Here's how the part is built. I have some questions about the finished solid (model axes, mm). A direction names the side the tool comes from. Round coordinates to 2 decimals unless told otherwise and drop trailing zeros. Loops run counter-clockwise (first coordinate to the right, second up) from the corner with the lowest first, then second, coordinate; pieces in that order, holes last. Notation, with made-up numbers: (26, 21.5) -> (47, 21.5) arc R16 ccw to (47, 28.5) -> close; hole circle Ø3 at (-11, 49.5). An arc over 180 degrees is marked (long way). Use one line per item in the form item = value. Start each with the question number.
Item 1: If we section it at D-D (y = 17.5): Write out the boundary of the cut face in (x, z), then the cut area to 3 significant figures.
Item 2: If we section it at A-A (x = 5.5): Write out the boundary of the cut face in (y, z), then the cut area to 3 significant figures.
Item 3: If we section it at B-B (y = 3): Write out the boundary of the cut face in (x, z), then the cut area to 3 significant figures.
Item 4: Thinking about a two-plate mould opening in Z: for faces 4 (the face through (5, 28, -10.5)), 5 (the face through (0, 13, 0)), 6 (the face through (7, 20, 16.5)), which applies, released by +Z, released by -Z, zero draft, split by the parting line, or undercut?
Item 5: If I drill on L1, parallel to Y at x = 7, z = -12.7; L2, parallel to Z at x = 6.5, y = 21.5; L3, parallel to Y at x = 7, z = 16, over which ranges is the centre line in solid material (lowest first)? Write a range as [from, to].
Item 6: I'm going to push flat-ended pins straight in: pin 1 Ø4 at (x, z) = (12.5, 12.5) entering from +Y; pin 2 Ø8 at (y, z) = (6, -8.5) entering from -X; pin 3 Ø5 at (x, y) = (7, 33) entering from -Z; pin 4 Ø3.5 at (x, z) = (11, 0) entering from +Y. Where does each tip first touch, or does it pass through?
Item 7: For faces 1 (the face through (7, 0, 0)), 2 (the face through (6.9, 29.7, 15.5)), 3 (the face through (7, 15, 0)), which set-ups out of +Z, -Z, +X, -X, +Y, -Y let a thin tool reach every point of the face, with its end or its side?
Item 8: If we section it at C-C (x = 3): Write out the boundary of the cut face in (y, z), then the cut area to 3 significant figures.
```python
from build123d import *

# Parameters (mm, degrees)
EXTRUDE_1_DEPTH     = 14
FILLET_1_R          = 7
CUT_EXTRUDE_START   = -1
SKETCH_7_R          = 5
CUT_EXTRUDE_1_DEPTH = 31
SKETCH_8_R          = 3.1
CUT_EXTRUDE_2_DEPTH = 35
CUT_EXTRUDE_START_2 = 2
SKETCH_10_R         = 1.5
CUT_EXTRUDE_3_DEPTH = 20


with BuildPart() as part:
    # 草图4 → 凸台-拉伸1 (new body)
    with BuildSketch(Plane(origin=(0, 0, 0), x_dir=(0, 0, -1), z_dir=(1, 0, 0))):
        with BuildLine():
            Line((0, 0), (16.5, 0))
            Line((16.5, 0), (16.5, 40))
            Line((16.5, 40), (10.5, 40))
            Line((10.5, 40), (10.5, 20))
            ThreePointArc((10.5, 20), (9.035533906, 16.464466094), (5.5, 15))
            Line((5.5, 15), (-5.5, 15))
            ThreePointArc((-5.5, 15), (-9.035533906, 16.464466094), (-10.5, 20))
            Line((-10.5, 20), (-10.5, 40))
            Line((-10.5, 40), (-16.5, 40))
            Line((-16.5, 40), (-16.5, 0))
            Line((-16.5, 0), (0, 0))
        make_face()
    extrude(amount=EXTRUDE_1_DEPTH)

    # 圆角1
    fillet_1_edges = [part.edges().sort_by_distance(p)[0] for p in [
        (0, 40, 13.5),
        (0, 40, -13.5),
        (14, 40, -13.5),
        (14, 40, 13.5),
    ]]
    fillet(fillet_1_edges, radius=FILLET_1_R - 0.0001)  # a hair under: the kernel refuses the full size

    # 草图7 → 切除-拉伸1 (cut)
    with BuildSketch(Plane.XY.offset(16.5).offset(CUT_EXTRUDE_START)):
        with Locations((7, 33)):
            Circle(SKETCH_7_R)
    extrude(amount=-CUT_EXTRUDE_1_DEPTH, mode=Mode.SUBTRACT)

    # 草图8 → 切除-拉伸2 (cut)
    with BuildSketch(Plane.XY.offset(16.5)):
        with Locations((7, 33)):
            Circle(SKETCH_8_R)
    extrude(amount=-CUT_EXTRUDE_2_DEPTH, mode=Mode.SUBTRACT)

    # 草图10 → 切除-拉伸3 (cut)
    with BuildSketch(Plane(origin=(0, 15, 0), x_dir=(1, 0, 0), z_dir=(0, 1, 0)).offset(CUT_EXTRUDE_START_2)):
        with Locations(Location((3, 0, 0), (0, 0, 270))):
            Circle(SKETCH_10_R)
        with Locations(Location((11, 0, 0), (0, 0, 270))):
            Circle(SKETCH_10_R)
    extrude(amount=-CUT_EXTRUDE_3_DEPTH, mode=Mode.SUBTRACT)


solid = part.part
```
Values found:
q1.outline = (0, -16.5) -> (14, -16.5) -> (14, -9.83) -> (0, -9.83) -> close; (0, 9.83) -> (14, 9.83) -> (14, 16.5) -> (0, 16.5) -> close
q1.area = 187 mm2
q2.outline = (0, -16.5) -> (30.29, -16.5) -> (30.29, -15.5) -> (28.23, -15.5) -> (28.23, -10.5) -> (20, -10.5) arc R5 cw to (15, -5.5) -> (15, 5.5) arc R5 cw to (20, 10.5) -> (28.23, 10.5) -> (28.23, 15.5) -> (30.29, 15.5) -> (30.29, 16.5) -> (0, 16.5) -> close; (35.71, -16.5) -> (39.84, -16.5) -> (39.84, -10.5) -> (37.77, -10.5) -> (37.77, -15.5) -> (35.71, -15.5) -> close; (35.71, 15.5) -> (37.77, 15.5) -> (37.77, 10.5) -> (39.84, 10.5) -> (39.84, 16.5) -> (35.71, 16.5) -> close
q2.area = 698 mm2
q3.outline = (0, -16.5) -> (14, -16.5) -> (14, 16.5) -> (0, 16.5) -> close; hole circle Ø3 at (3, 0); hole circle Ø3 at (11, 0)
q3.area = 448 mm2
q4.face_4 = undercut
q4.face_5 = zero draft
q4.face_6 = released by +Z
q5.L1 = [0, 28], [38, 40]
q5.L2 = [-16.5, -10.5], [10.5, 16.5]
q5.L3 = [0, 29.9], [36.1, 40]
q6.pin_1 = 39.06
q6.pin_2 = 0
q6.pin_3 = through
q6.pin_4 = 15
q7.face_1 = +Z, -Z, +X, -X, -Y
q7.face_2 = none
q7.face_3 = +X, -X, +Y
q8.outline = (0, -16.5) -> (38.74, -16.5) -> (38.74, -10.5) -> (36, -10.5) -> (36, -15.5) -> (30, -15.5) -> (30, -10.5) -> (20, -10.5) arc R5 cw to (15, -5.5) -> (15, -1.5) -> (0, -1.5) -> close; (0, 1.5) -> (15, 1.5) -> (15, 5.5) arc R5 cw to (20, 10.5) -> (30, 10.5) -> (30, 15.5) -> (36, 15.5) -> (36, 10.5) -> (38.74, 10.5) -> (38.74, 16.5) -> (0, 16.5) -> close
q8.area = 686 mm2
